For this review, take the finished solid that the model builds, in its own axes (mm). Face numbers are marked on the shaded views. A direction names the side the tool comes from. Coordinates: 2 decimals unless noted, no trailing zeros. Write each loop counter-clockwise with the first axis right and the second up, starting at its lowest first coordinate (ties: lowest second). Pieces come first, ordered by that corner, then holes. Notation, with made-up numbers: (2, 7.25) - (25, 7.25) arc R32 ccw to (25, 39.25) - close; hole circle Ø7 at (40.5, 19.5). An arc over 180 degrees is marked (long way). Use one line per item in the form item = value. Start each with the question number.
1) Mouldability with a two-part tool opening along X and no side actions: class the marked faces 3, 4 and 5 as pulls with the +X half, pulls with the -X half, needs draft (parallel to the pull), parting line crosses it, or undercut.
2) We need section A-A (x = 52.5). Give the boundary of the cut face in (y, z).
3) Insertion check: P1, Ø4.5, axis at y = 0, z = 0, coming from the -X side; P2, Ø1, axis at x = 26.5, y = 13.5, coming from the +Z side; P3, Ø8, axis at x = 27.5, y = 11, coming from the +Z side; P4, Ø5, axis at x = 23.5, y = 10, coming from the -Z side. Each pin has a flat end and moves straight along its axis. Give the tip position at first contact, or say it passes through.
4) We need section B-B (x = 32). Give the boundary of the cut face in (y, z).
5) Tool access review of the marked faces 1 and 2: name each direction out of +Z, -Z, +X, -X, +Y, -Y from which nothing blocks a thin tool from reaching the whole face with its end or side.
6) For L1, parallel to X at y = 17, z = -0.5; L2, parallel to Y at x = 40, z = 0; L3, parallel to Z at x = 72, y = -2, list the stretches that pass through material, from the lowest coordinate up. Write a range as from..to.
```python
from build123d import *

# Parameters (mm, degrees)
FILLET1_R                   = 1
M6_TAPPED_HOLE1_D           = 5
M6_TAPPED_HOLE1_CSINK_D     = 6.05
M6_TAPPED_HOLE1_CSINK_ANGLE = 90


# Read off the part's stored shape, not the designer's step: Revolve1
with BuildPart() as part:
    # Revolve1 outline → Revolve1 (revolve)
    with BuildSketch(Plane.YX):
        Polygon((0, 80), (0, 0), (17.5, 0), (17.5, 3.5), (16.1, 3.5), (16.1, 5), (17.61, 5), (17.5, 45), (19, 45), (19, 50), (15, 50), (15, 70), (13.95, 70), (13.95, 71.5), (15, 71.5), (15, 80), align=None)
    revolve(axis=Axis((0, 0, 0), (1, 0, 0)))

    # Fillet1
    fillet1_edges = [part.edges().sort_by_distance(p)[0] for p in [
        (50, -15, 0),
    ]]
    fillet(fillet1_edges, radius=FILLET1_R)

    # M6 Tapped Hole1 (through all)
    with Locations(Plane(origin=(80, 0, 0), x_dir=(0, 0, 1), z_dir=(1, 0, 0))):
        with Locations((0, 0)):
            CounterSinkHole(M6_TAPPED_HOLE1_D / 2, M6_TAPPED_HOLE1_CSINK_D / 2, counter_sink_angle=M6_TAPPED_HOLE1_CSINK_ANGLE)


solid = part.part
```
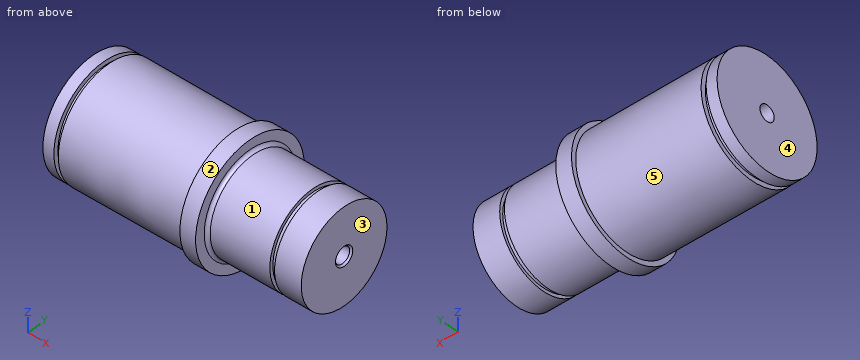
Determined:
q1.face_3 = pulls with the +X half
q1.face_4 = pulls with the -X half
q1.face_5 = undercut
q2.outline = circle Ø30 at (0, 0); hole circle Ø5 at (0, 0)
q3.P1 = through
q3.P2 = 11.79
q3.P3 = 16.09
q3.P4 = -15.88
q4.outline = circle Ø35.07 at (0, 0); hole circle Ø5 at (0, 0)
q5.face_1 = +X
q5.face_2 = +X, -X
q6.L1 = 0..3.5, 5..50
q6.L2 = -17.51..-2.5, 2.5..17.51
q6.L3 = -14.87..-1.5, 1.5..14.87
